Autodesk Inventor part; units mm, degrees
ref_plane "YZ Plane" through (0, 0, 0) normal (1, 0, 0) x (0, 1, 0)
ref_plane "XZ Plane" through (0, 0, 0) normal (0, 1, 0) x (-1, 0, 0)
ref_plane "XY Plane" through (0, 0, 0) normal (0, 0, 1) x (1, 0, 0)
sketch "Sketch1" plane through (0, 0, 0) normal (0, 0, 1) x (1, 0, 0)
  line L0 (0, 0) -> (-13, 0)
  line L1 (-13, 0) -> (-13, 3.1)
  line L2 (-12.8, 3.3) -> (-10.5, 3.3)
  line L3 (-10.5, 3.3) -> (-10.5, 2.3)
  line L4 (-10.5, 2.3) -> (-2.5, 2.3)
  line L5 (-2.5, 2.3) -> (-2.5, 3.3)
  line L6 (-2.5, 3.3) -> (-0.2, 3.3)
  line L7 (0, 3.1) -> (0, 0)
  arc A0 (-12.8, 3.3) -> (-13, 3.1) centre (-12.8, 3.1) ccw
  arc A1 (0, 3.1) -> (-0.2, 3.3) centre (-0.2, 3.1) ccw
  line L8 (-10.5, 2.3) -> (-10.5, 0)
  line L9 (-2.5, 2.3) -> (-2.5, 0)
  point P0 (-13, 3.3)
  point P1 (0, 3.3)
  dimension "d0" = 13
  dimension "d1" = 3.3
  dimension "d2" = 2.5
  dimension "d3" = 1
  dimension "d5" = 8
  dimension "d6" = 1
  dimension "d7" = 2.5
  dimension "d8" = 0.2
revolve "Revolution1" add sketch "Sketch1" angle 360 about axis through (0, 0, 0) along (-1, 0, 0)
ref_plane "Work Plane1" through (0, 0, 0) normal (1, 0, 0) x (0, 0, -1)
sketch "Sketch2" plane through (0, 0, 0) normal (1, 0, 0) x (0, 0, -1)
  circle A0 centre (0, 0) radius 0.3
  dimension "d11" = 0.6
sketch "Sketch3" plane through (0, 0, 0) normal (0, 0, 1) x (1, 0, 0)
  line L0 (0, 0) -> (12.3, 0)
  line L1 (12.5, -0.2) -> (12.5, -12.5)
  arc A0 (12.5, -0.2) -> (12.3, 0) centre (12.3, -0.2) ccw
  point P0 (12.5, 0)
  dimension "d12" = 12.5
  dimension "d13" = 12.5
  dimension "d14" = 0.2
sweep "Sweep1" add profiles "Sketch2" path "Sketch3"
ref_plane "Work Plane2" through (-13, 0, 0) normal (-1, 0, 0) x (0, 0, 1)
sketch "Sketch4" plane through (-13, 0, 0) normal (-1, 0, 0) x (0, 0, 1)
  circle A0 centre (0, 0) radius 0.3
  circle A1 centre (0, 0) radius 0.3
  point P0 (0, 0)
  dimension "d18" = 0.6
sketch "Sketch5" plane through (0, 0, 0) normal (0, 0, 1) x (1, 0, 0)
  line L0 (-13, 3.1) -> (-13, -3.1)
  line L1 (-13, 0) -> (-25.3, 0)
  line L2 (-25.5, -0.2) -> (-25.5, -12.5)
  arc A0 (-25.3, 0) -> (-25.5, -0.2) centre (-25.3, -0.2) ccw
  point P0 (0, 0)
  point P1 (-25.5, 0)
  dimension "d19" = 12.5
  dimension "d20" = 12.5
  dimension "d21" = 0.2
sweep "Sweep2" add profiles "Sketch4" path "Sketch5" path curves L1 A0 L2
equation "\"BendRadius\" = Thickness"
equation "\"BendReliefWidth\" = Thickness"
equation "\"BendReliefDepth\" = 0.5 * Thickness"
equation "\"CornerReliefSize\" = 4 * Thickness"
equation "\"MinimumRemnant\" = 2 * Thickness"
equation "\"TransitionRadius\" = BendRadius"
equation "\"JacobiRadiusSize\" = BendRadius"
equation "\"GapSize\" = Thickness"
properties part number "A44"
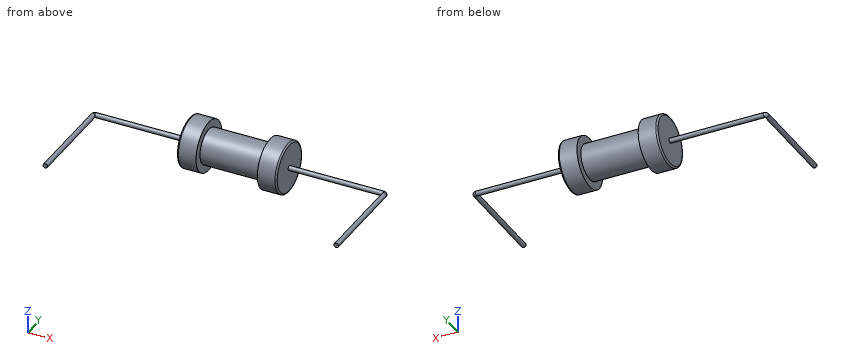
Build history of the part. All positions in model axes, mm. Give positions to 0.01 mm unless a question says otherwise; leave off trailing zeros. Loops run counter-clockwise (first coordinate to the right, second up) from the corner with the lowest first, then second, coordinate; pieces in that order, holes last.
Item 1: Drill centre lines: line 1 (X direction, y = -2.25, z = 1.75); line 2 (Y direction, x = -11, z = 0); line 3 (Y direction, x = -5.5, z = -0.75). Where is each one in solid material? Low to high.
Answers follow:
line 1: x = -13 to -10.5, -2.5 to 0
line 2: y = -3.3 to 3.3
line 3: y = -2.17 to 2.17
Item 2: Flat gauge pins, fed straight in: pin 1 (2 mm diameter, centred on y = -1.5, z = -2.5, fed in from +X); pin 2 (1 mm diameter, centred on x = -1, z = -1, fed in from +Y); pin 3 (1 mm diameter, centred on x = 7, z = 2.5, fed in from -Y); pin 4 (2 mm diameter, centred on y = 0.5, z = 1.5, fed in from -X). Where does each tip first touch, or does it go through?
Answers follow:
pin 1: stops at x = 0
pin 2: stops at y = 3.26
pin 3: passes through
pin 4: stops at x = -13
Item 3: Slice it at D-D, the plane x = 6.5. List the corners of the cut face in (y, z), and give its area (3 significant figures).
Answers follow:
outline: circle Ø0.6 at (0, 0)
area: 0.283 mm2
Item 4: Slice it at A-A, the plane y = -4.5. List the corners of the cut face in (x, z).
Answers follow:
outline: circle Ø0.6 at (-25.5, 0); circle Ø0.6 at (12.5, 0)
Item 5: Slice it at B-B, the plane x = -1. List the corners of the cut face in (y, z).
Answers follow:
outline: circle Ø6.6 at (0, 0)
Item 6: Slice it at C-C, the plane y = -0.75. Give the number of separate pieces and of enclosed holes in the cut face, and give its area (3 significant figures).
Answers follow:
separate pieces: 3
enclosed holes: 0
area: 67.5 mm2
